Here's how the part is built. I have some questions about the finished solid (model axes, mm). Face numbers are marked on the shaded views. A direction names the side the tool comes from. Coordinates: 2 decimals unless noted, no trailing zeros. Write each loop counter-clockwise with the first axis right and the second up, starting at its lowest first coordinate (ties: lowest second). Pieces come first, ordered by that corner, then holes. Notation, with made-up numbers: (81, -30) -> (124, -30) arc R20 cw to (124, -7) -> close; hole circle Ø5 at (-10.75, 2). An arc over 180 degrees is marked (long way). Put each result on its own line as item: value.
```python
from build123d import *

# Parameters (mm, degrees)
BASE_FLANGE1_DEPTH     = 1
SKETCHED_START         = -30
SKETCHED_BEND5_DEPTH   = 60
SKETCHED_BEND5_2_DEPTH = 15
SKETCHED_START_2       = 15
SKETCHED_BEND5_3_DEPTH = 15
SKETCHED_BEND5_4_DEPTH = 60
SKETCHED_START_3       = -15
SKETCHED_BEND5_5_DEPTH = 30
SKETCHED_BEND6_DEPTH   = 60
SKETCHED_BEND6_2_DEPTH = 15
SKETCHED_BEND6_3_DEPTH = 15
SKETCHED_BEND6_4_DEPTH = 30
SKETCHED_BEND6_5_DEPTH = 60
SKETCHED_START_4       = -28.356310605
SKETCHED_BEND7_DEPTH   = 23
SKETCHED_BEND7_2_DEPTH = 23
SKETCHED_START_5       = 11.547743288
SKETCHED_BEND8_DEPTH   = 70
SKETCHED_BEND8_2_DEPTH = 70
CUT_EXTRUDE1_DEPTH     = 10
F_6_CLEARANCE_HOLE4_D  = 3.7973
F_6_CLEARANCE_HOLE2_D  = 3.7973
F_3_0MM_DOWEL_HOLE1_D  = 3
SKETCH47_R             = 1.525
CUT_EXTRUDE2_DEPTH     = 10
CUT_EXTRUDE3_DEPTH     = 10
FILLET2_R              = 13
FILLET1_R              = 1


# Read off the part's stored shape, not the designer's step: Sketched Bend5, Sketched Bend6, Sketched Bend7, Sketched Bend8
# Sheet-metal steps are written as plain solids
with BuildPart() as part:
    # Sketch1 → Base-Flange1 (new body)
    with BuildSketch(Plane.XY):
        Polygon((-30, -30.5), (-15, -30.5), (-15, -69.5), (15, -69.5), (15, -30.5), (30, -30.5), (30, -7.5), (15, -7.5), (15, 15.5), (30, 15.5), (30, 85.5), (-30, 85.5), (-30, 15.5), (-15, 15.5), (-15, -7.5), (-30, -7.5), align=None)
    extrude(amount=-BASE_FLANGE1_DEPTH)

    # Sketched Bend5 outline → Sketched Bend5 (cut)
    with BuildSketch(Plane.YZ.offset(SKETCHED_START)):
        with BuildLine():
            Line((15.714213562, -0.585786438), (16.128427124, -1))
            Line((16.128427124, -1), (85.5, -1))
            Line((85.5, -1), (85.5, 0))
            Line((85.5, 0), (14.3, 0))
            ThreePointArc((14.3, 0), (15.065366865, -0.152240935), (15.714213562, -0.585786438))
        make_face()
    extrude(amount=SKETCHED_BEND5_DEPTH, mode=Mode.SUBTRACT)

    # Sketched Bend5 2 outline → Sketched Bend5 2 (cut)
    with BuildSketch(Plane.YZ.offset(SKETCHED_START)):
        with BuildLine():
            Line((15.729701149, -0.601274024), (15.714213562, -0.585786438))
            ThreePointArc((15.714213562, -0.585786438), (15.610403483, -0.48909209), (15.5, -0.4))
            Line((15.5, -0.4), (15.5, -0.830975173))
            Line((15.5, -0.830975173), (15.729701149, -0.601274024))
        make_face()
    extrude(amount=SKETCHED_BEND5_2_DEPTH, mode=Mode.SUBTRACT)

    # Sketched Bend5 3 outline → Sketched Bend5 3 (cut)
    with BuildSketch(Plane.YZ.offset(SKETCHED_START_2)):
        with BuildLine():
            Line((15.729701149, -0.601274024), (15.714213562, -0.585786438))
            ThreePointArc((15.714213562, -0.585786438), (15.610403483, -0.48909209), (15.5, -0.4))
            Line((15.5, -0.4), (15.5, -0.830975173))
            Line((15.5, -0.830975173), (15.729701149, -0.601274024))
        make_face()
    extrude(amount=SKETCHED_BEND5_3_DEPTH, mode=Mode.SUBTRACT)

    # Sketched Bend5 4 outline → Sketched Bend5 4 (add)
    with BuildSketch(Plane.YZ.offset(SKETCHED_START)):
        Polygon((65.227175832, -50.098748707), (16.128427124, -1), (15.5, -1), (15.5, -0.830975173), (15.022594368, -1.308380805), (64.520069051, -50.805855488), align=None)
    extrude(amount=SKETCHED_BEND5_4_DEPTH)

    # Sketched Bend5 5 outline → Sketched Bend5 5 (add)
    with BuildSketch(Plane.YZ.offset(SKETCHED_START_3)):
        with BuildLine():
            Line((15.022594368, -1.308380805), (15.330975173, -1))
            Line((15.330975173, -1), (14.3, -1))
            ThreePointArc((14.3, -1), (14.682683432, -1.076120467), (15.007106781, -1.292893219))
            Line((15.007106781, -1.292893219), (15.022594368, -1.308380805))
        make_face()
    extrude(amount=SKETCHED_BEND5_5_DEPTH)

    # Sketched Bend6 outline → Sketched Bend6 (cut)
    with BuildSketch(Plane.YZ.offset(SKETCHED_START)):
        with BuildLine():
            ThreePointArc((-5.710951377, -1), (-6.476318242, -0.847759065), (-7.12516494, -0.414213562))
            Line((-7.12516494, -0.414213562), (-7.539378502, 0))
            Line((-7.539378502, 0), (-69.5, 0))
            Line((-69.5, 0), (-69.5, -1))
            Line((-69.5, -1), (-5.710951377, -1))
        make_face()
    extrude(amount=SKETCHED_BEND6_DEPTH, mode=Mode.SUBTRACT)

    # Sketched Bend6 2 outline → Sketched Bend6 2 (cut)
    with BuildSketch(Plane.YZ.offset(SKETCHED_START)):
        Polygon((-7.539378502, 0), (-7.5, -0.039378502), (-7.5, 0), align=None)
    extrude(amount=SKETCHED_BEND6_2_DEPTH, mode=Mode.SUBTRACT)

    # Sketched Bend6 3 outline → Sketched Bend6 3 (cut)
    with BuildSketch(Plane.YZ.offset(SKETCHED_START_2)):
        Polygon((-7.539378502, 0), (-7.5, -0.039378502), (-7.5, 0), align=None)
    extrude(amount=SKETCHED_BEND6_3_DEPTH, mode=Mode.SUBTRACT)

    # Sketched Bend6 4 outline → Sketched Bend6 4 (add)
    with BuildSketch(Plane.YZ.offset(SKETCHED_START_3)):
        with BuildLine():
            Line((-7.539378502, 0), (-5.710951377, 0))
            ThreePointArc((-5.710951377, 0), (-6.09363481, 0.076120467), (-6.418058159, 0.292893219))
            Line((-6.418058159, 0.292893219), (-50.690686454, 44.565521514))
            Line((-50.690686454, 44.565521514), (-51.397793235, 43.858414733))
            Line((-51.397793235, 43.858414733), (-7.539378502, 0))
        make_face()
    extrude(amount=SKETCHED_BEND6_4_DEPTH)

    # Sketched Bend6 5 outline → Sketched Bend6 5 (add)
    with BuildSketch(Plane.YZ.offset(SKETCHED_START)):
        Polygon((-23.820628769, 16.281250267), (-7.557172802, 0.0177943), (-6.850066021, 0.724901081), (-23.113521988, 16.988357048), align=None)
    extrude(amount=SKETCHED_BEND6_5_DEPTH)

    # Sketched Bend7 outline → Sketched Bend7 (cut)
    with BuildSketch(Plane(origin=(0, 0, 0), x_dir=(1, 0, 0), z_dir=(0, 0.707106781186546, -0.707106781186549)).offset(SKETCHED_START_4)):
        with BuildLine():
            ThreePointArc((-16.732050807, 4.331145665), (-16, 5.063196472), (-15, 5.331145665))
            Line((-15, 5.331145665), (-30, 5.331145665))
            Line((-30, 5.331145665), (-30, 4.331145665))
            Line((-30, 4.331145665), (-16.732050807, 4.331145665))
        make_face()
        with BuildLine():
            Line((30, 5.331145665), (15, 5.331145665))
            ThreePointArc((15, 5.331145665), (16, 5.063196472), (16.732050807, 4.331145665))
            Line((16.732050807, 4.331145665), (30, 4.331145665))
            Line((30, 4.331145665), (30, 5.331145665))
        make_face()
    extrude(amount=SKETCHED_BEND7_DEPTH, mode=Mode.SUBTRACT)

    # Sketched Bend7 2 outline → Sketched Bend7 2 (add)
    with BuildSketch(Plane(origin=(0, 0, 0), x_dir=(1, 0, 0), z_dir=(0, 0.707106781186546, -0.707106781186549)).offset(SKETCHED_START_4)):
        with BuildLine():
            Line((-15, 4.331145665), (-16.732050807, 4.331145665))
            ThreePointArc((-16.732050807, 4.331145665), (-16.931851652, 3.848783755), (-17, 3.331145665))
            Line((-17, 3.331145665), (-17, -9.312659845))
            Line((-17, -9.312659845), (-16, -9.312659845))
            Line((-16, -9.312659845), (-16, 3.331145665))
            ThreePointArc((-16, 3.331145665), (-15.707106781, 4.038252446), (-15, 4.331145665))
        make_face()
        with BuildLine():
            ThreePointArc((17, 3.331145665), (16.931851652, 3.848783755), (16.732050807, 4.331145665))
            Line((16.732050807, 4.331145665), (15, 4.331145665))
            ThreePointArc((15, 4.331145665), (15.707106781, 4.038252446), (16, 3.331145665))
            Line((16, 3.331145665), (16, -9.312659845))
            Line((16, -9.312659845), (17, -9.312659845))
            Line((17, -9.312659845), (17, 3.331145665))
        make_face()
    extrude(amount=SKETCHED_BEND7_2_DEPTH)

    # Sketched Bend8 outline → Sketched Bend8 (cut)
    with BuildSketch(Plane(origin=(0, 0, 0), x_dir=(1, 0, 0), z_dir=(0, 0.707106781186546, -0.707106781186549)).offset(SKETCHED_START_5)):
        with BuildLine():
            Line((-30, -10.697413409), (-16.732050808, -10.697413409))
            ThreePointArc((-16.732050808, -10.697413409), (-16, -9.965362601), (-15, -9.697413409))
            Line((-15, -9.697413409), (-30, -9.697413409))
            Line((-30, -9.697413409), (-30, -10.697413409))
        make_face()
        with BuildLine():
            Line((30, -9.697413409), (15, -9.697413409))
            ThreePointArc((15, -9.697413409), (16, -9.965362601), (16.732050808, -10.697413409))
            Line((16.732050808, -10.697413409), (30, -10.697413409))
            Line((30, -10.697413409), (30, -9.697413409))
        make_face()
    extrude(amount=SKETCHED_BEND8_DEPTH, mode=Mode.SUBTRACT)

    # Sketched Bend8 2 outline → Sketched Bend8 2 (add)
    with BuildSketch(Plane(origin=(0, 0, 0), x_dir=(1, 0, 0), z_dir=(0, 0.707106781186546, -0.707106781186549)).offset(SKETCHED_START_5)):
        with BuildLine():
            ThreePointArc((-16.732050808, -10.697413409), (-16.931851653, -11.179775319), (-17, -11.697413409))
            Line((-17, -11.697413409), (-17, -24.341218918))
            Line((-17, -24.341218918), (-16, -24.341218918))
            Line((-16, -24.341218918), (-16, -11.697413409))
            ThreePointArc((-16, -11.697413409), (-15.707106781, -10.990306628), (-15, -10.697413409))
            Line((-15, -10.697413409), (-16.732050808, -10.697413409))
        make_face()
        with BuildLine():
            Line((16.732050808, -10.697413409), (15, -10.697413409))
            ThreePointArc((15, -10.697413409), (15.707106781, -10.990306628), (16, -11.697413409))
            Line((16, -11.697413409), (16, -24.341218918))
            Line((16, -24.341218918), (17, -24.341218918))
            Line((17, -24.341218918), (17, -11.697413409))
            ThreePointArc((17, -11.697413409), (16.931851653, -11.179775319), (16.732050808, -10.697413409))
        make_face()
    extrude(amount=SKETCHED_BEND8_2_DEPTH)

    # Sketch36 → Cut-Extrude1 (cut)
    with BuildSketch(Plane(origin=(0, 7.564213562, 7.564213562), x_dir=(1, 0, 0), z_dir=(0, 0.7071067811865487, 0.7071067811865465))):
        with BuildLine():
            Line((-9, 28), (9, 28))
            ThreePointArc((9, 28), (12, 25), (9, 22))
            Line((9, 22), (-9, 22))
            ThreePointArc((-9, 22), (-12, 25), (-9, 28))
        make_face()
        with BuildLine():
            Line((-9, 41), (9, 41))
            ThreePointArc((9, 41), (12, 38), (9, 35))
            Line((9, 35), (-9, 35))
            ThreePointArc((-9, 35), (-12, 38), (-9, 41))
        make_face()
        with BuildLine():
            Line((-9, 54), (9, 54))
            ThreePointArc((9, 54), (12, 51), (9, 48))
            Line((9, 48), (-9, 48))
            ThreePointArc((-9, 48), (-12, 51), (-9, 54))
        make_face()
        with BuildLine():
            Line((-9, 73), (9, 73))
            ThreePointArc((9, 73), (12, 70), (9, 67))
            Line((9, 67), (-9, 67))
            ThreePointArc((-9, 67), (-12, 70), (-9, 73))
        make_face()
    extrude(amount=-CUT_EXTRUDE1_DEPTH, mode=Mode.SUBTRACT)

    # #6 Clearance Hole4 (through all)
    with Locations(Plane(origin=(0, 7.564213562, 7.564213562), x_dir=(1, 0, 0), z_dir=(0, 0.7071067811865487, 0.7071067811865465))):
        with Locations((-8.5, 18.025840533), (8.5, 18.025840533), (0, -14.745359227), (-8.5, -36.745359227), (8.5, -36.745359227)):
            Hole(F_6_CLEARANCE_HOLE4_D / 2)

    # #6 Clearance Hole2 (through all)
    with Locations(Plane(origin=(17, 0, 0), x_dir=(0, 0, -1), z_dir=(1, 0, 0))):
        with Locations((-9.311868306, -5.334166607), (-16.382936118, -12.405234419), (-0.914625389, 24.316668374), (6.156442422, 31.387736186)):
            Hole(F_6_CLEARANCE_HOLE2_D / 2)

    # Ø3.0mm Dowel Hole1 (through all)
    with Locations(Plane(origin=(0, 7.564213562, 7.564213562), x_dir=(1, 0, 0), z_dir=(0, 0.7071067811865487, 0.7071067811865465))):
        with Locations((0, 61.187743288)):
            Hole(F_3_0MM_DOWEL_HOLE1_D / 2)

    # Sketch47 → Cut-Extrude2 (cut)
    with BuildSketch(Plane(origin=(0, -3.06258247, -3.06258247), x_dir=(1, 0, 0), z_dir=(0, 0.7071067811865487, 0.7071067811865465))):
        with Locations(Location((0, -54.856310605, 0), (0, 0, 270))):
            Circle(SKETCH47_R)
    extrude(amount=-CUT_EXTRUDE2_DEPTH, mode=Mode.SUBTRACT)

    # Sketch48 → Cut-Extrude3 (cut)
    with BuildSketch(Plane.XY):
        Polygon((-10, 10.8), (10, 10.8), (5, 5.8), (-5, 5.8), align=None)
        Polygon((-10, -2.210951377), (-5, 2.789048623), (5, 2.789048623), (10, -2.210951377), align=None)
    extrude(amount=-CUT_EXTRUDE3_DEPTH, mode=Mode.SUBTRACT)

    # Fillet2
    fillet2_edges = [part.edges().sort_by_distance(p)[0] for p in [
        (-15, -51.044239844, 44.211968124),
        (15, -51.044239844, 44.211968124),
    ]]
    fillet(fillet2_edges, radius=FILLET2_R)

    # Fillet1
    fillet1_edges = [part.edges().sort_by_distance(p)[0] for p in [
        (-16.5, -13.465894591, 26.635984446),
        (-16.5, 2.797561376, 10.372528478),
        (16.5, 2.797561376, 10.372528478),
        (16.5, -13.465894591, 26.635984446),
        (-16.5, 25.377328546, 9.046353373),
        (-16.5, 74.874803229, -40.45112131),
        (16.5, 74.874803229, -40.45112131),
        (16.5, 25.377328546, 9.046353373),
        (-5, 5.8, -0.5),
        (-10, 10.8, -0.5),
        (10, 10.8, -0.5),
        (5, 5.8, -0.5),
        (10, -2.210951377, -0.5),
        (-10, -2.210951377, -0.5),
        (-5, 2.789048623, -0.5),
        (5, 2.789048623, -0.5),
    ]]
    fillet(fillet1_edges, radius=FILLET1_R)


solid = part.part
```
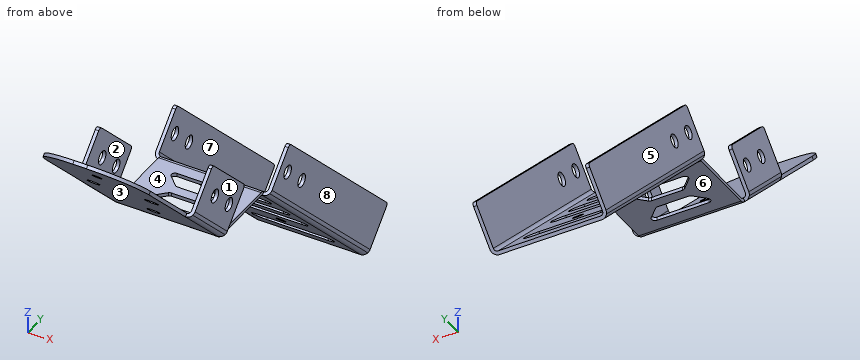
Item 1: For P1, Ø1.6, axis at y = -1, z = -0.5, coming from the +X side; P2, Ø1.5, axis at x = 1, z = -13, coming from the +Y side; P3, Ø2.5, axis at y = -5.33, z = 9.31, coming from the +X side; P4, Ø0.8, axis at x = 2, z = -0.5, coming from the +Y side, each with a flat end and sliding along its axis, tell me the tip position at first contact or that it passes through.
Output:
P1: stops at x = 15
P2: stops at y = 28.88
P3: passes through
P4: stops at y = 16.03
Item 2: Imagine slicing it at A-A on y = -33. Write out the boundary of the cut face in (x, z).
Output:
outline: (-15, 25.46) -> (15, 25.46) -> (15, 26.87) -> (-15, 26.87) -> close
Item 3: Which directions (+Z, -Z, +X, -X, +Y, -Y) give clear straight access to the entire face, cutting with the end or side of a thin tool? Please do the marked faces 4, 5, 6, 7 and 8.
Output:
face 4: +Z, +X, -X, +Y
face 5: +Z, -Z, -X, +Y, -Y
face 6: -Z, +X, -X, -Y
face 7: +Z, +Y
face 8: +Z, -Z, +X, +Y, -Y
Item 4: If we mould it in two halves opening along X, with no side actions, what happens to the marked faces 1, 2 and 3? For each: released by +X, released by -X, zero draft, split by the parting line, or undercut.
Output:
face 1: released by +X
face 2: undercut
face 3: zero draft
Item 5: Please list where these lines run through material, in increasing order: line 1 along X through (y, z) = (-10.5, 6); line 2 along Z through (x, y) = (-10.5, -41.5); line 3 along Z through (x, y) = (12, -1.5). Write a range as from..to.
Output:
line 1: x = -17..-16, 16..17
line 2: z = 33.96..35.37
line 3: z = -1..0
